Model file for the job. Use its own axes, mm. Give positions to 0.01 mm unless a question says otherwise; leave off trailing zeros. Loops run counter-clockwise (first coordinate to the right, second up) from the corner with the lowest first, then second, coordinate; pieces in that order, holes last. Notation, with made-up numbers: (1, 81.25) -> (18, 81.25) arc R18 ccw to (18, 112.25) -> close; hole circle Ø11 at (88.25, 5.25). An arc over 180 degrees is marked (long way). Use CSV: the item, a comma, the result in double quotes. Start each with the question number.
(1) Cut at B-B on y = 0. Write the cut outline in (x, z).
(2) Cut at D-D on x = 57. Write the cut outline in (y, z), then the cut area to 3 significant figures.
(3) Cut at C-C on y = -34.5. Write the cut outline in (x, z).
(4) Cut at A-A on x = 28. Write the cut outline in (y, z).
(5) Flat gauge pins, fed straight in: pin 1 (2 mm diameter, centred on x = 54, y = -12, fed in from -Z); pin 2 (3.5 mm diameter, centred on x = 57, y = 27.5, fed in from -Z). Where does each tip first touch, or does it go through?
(6) Drill centre lines: probe 1 along Y at (x, z) = (36, 2.25); probe 2 along Y at (x, z) = (57, 1.1); probe 3 along Y at (x, z) = (24, 1.55). Where is each one in solid material? Low to high.
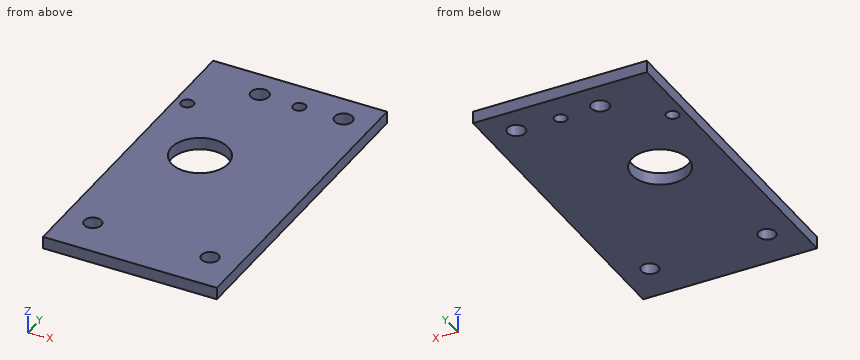
from build123d import *

# Parameters (mm, degrees)
SKETCH_1_W                = 40
SKETCH_1_H                = 29
EXTRUDE_1_DEPTH           = 3
CUT_EXTRUDE_1_DEPTH       = 3
SKETCH_3_W                = 40
SKETCH_3_H                = 3
EXTRUDE_2_DEPTH           = 10
SKETCH_4_W                = 40
SKETCH_4_H                = 3
EXTRUDE_3_DEPTH           = 10
SKETCH_6_W                = 3
SKETCH_6_H                = 49
EXTRUDE_5_DEPTH           = 42
SKETCH_8_W                = 3
SKETCH_8_H                = 49
EXTRUDE_6_DEPTH           = 2
SKETCH_9_W                = 3
SKETCH_9_H                = 49
EXTRUDE_7_DEPTH           = 2
SKETCH_10_W               = 86
SKETCH_10_H               = 3
EXTRUDE_8_DEPTH           = 10
SKETCH_11_W               = 86
SKETCH_11_H               = 3
EXTRUDE_9_DEPTH           = 10
SKETCH_7_R                = 7
CUT_EXTRUDE_4_DEPTH       = 10
SKETCH_14_W               = 3
SKETCH_14_H               = 69
CUT_EXTRUDE_5_DEPTH       = 43
SKETCH_17_W               = 43
SKETCH_17_H               = 3
EXTRUDE_10_DEPTH          = 20
SKETCH_18_R               = 2.1
CUT_EXTRUDE_6_DEPTH       = 10
SKETCH_20_W               = 43
SKETCH_20_H               = 3
EXTRUDE_11_DEPTH          = 10
SKETCH_21_W               = 43
SKETCH_21_H               = 3
CUT_EXTRUDE_7_DEPTH       = 20
SKETCH_24_R               = 2.2
CUT_EXTRUDE_8_DEPTH       = 30
SKETCH_25_R               = 1.55
CUT_EXTRUDE_11_DEPTH      = 1
CUT_EXTRUDE_11_DEPTH_BACK = 4


with BuildPart() as part:
    # ｽｹｯﾁ1 → ﾎﾞｽ - 押し出し1 (new body)
    with BuildSketch(Plane.XY):
        Rectangle(SKETCH_1_W, SKETCH_1_H)
    extrude(amount=EXTRUDE_1_DEPTH)

    # ｽｹｯﾁ2 → ｶｯﾄ - 押し出し1 (cut)
    with BuildSketch(Plane.XY.offset(3)):
        with BuildLine():
            ThreePointArc((-14.4, 10.5), (-15.01507576, 11.98492424), (-16.5, 12.6))
            Line((-16.5, 12.6), (-16.5, 10.5))
            Line((-16.5, 10.5), (-18.6, 10.5))
            ThreePointArc((-18.6, 10.5), (-16.5, 8.4), (-14.4, 10.5))
        make_face()
        with BuildLine():
            Line((-16.5, 10.5), (-16.5, 12.6))
            ThreePointArc((-16.5, 12.6), (-17.98492424, 11.98492424), (-18.6, 10.5))
            Line((-18.6, 10.5), (-16.5, 10.5))
        make_face()
        with BuildLine():
            ThreePointArc((-18.6, -10.5), (-17.98492424, -11.98492424), (-16.5, -12.6))
            Line((-16.5, -12.6), (-16.5, -10.5))
            Line((-16.5, -10.5), (-18.6, -10.5))
        make_face()
        with BuildLine():
            Line((-16.5, -10.5), (-16.5, -12.6))
            ThreePointArc((-16.5, -12.6), (-15.01507576, -11.98492424), (-14.4, -10.5))
            ThreePointArc((-14.4, -10.5), (-16.5, -8.4), (-18.6, -10.5))
            Line((-18.6, -10.5), (-16.5, -10.5))
        make_face()
        with BuildLine():
            ThreePointArc((18.6, -10.5), (15.01507576, -9.01507576), (16.5, -12.6))
            Line((16.5, -12.6), (16.5, -10.5))
            Line((16.5, -10.5), (18.6, -10.5))
        make_face()
        with BuildLine():
            Line((16.5, -10.5), (16.5, -12.6))
            ThreePointArc((16.5, -12.6), (17.98492424, -11.98492424), (18.6, -10.5))
            Line((18.6, -10.5), (16.5, -10.5))
        make_face()
        with BuildLine():
            ThreePointArc((18.6, 10.5), (17.98492424, 11.98492424), (16.5, 12.6))
            Line((16.5, 12.6), (16.5, 10.5))
            Line((16.5, 10.5), (18.6, 10.5))
        make_face()
        with BuildLine():
            Line((16.5, 10.5), (16.5, 12.6))
            ThreePointArc((16.5, 12.6), (15.01507576, 9.01507576), (18.6, 10.5))
            Line((18.6, 10.5), (16.5, 10.5))
        make_face()
    extrude(amount=-CUT_EXTRUDE_1_DEPTH, mode=Mode.SUBTRACT)

    # ｽｹｯﾁ3 → ﾎﾞｽ - 押し出し2 (add)
    with BuildSketch(Plane.XZ.offset(14.5)):
        with Locations((0, 1.5)):
            Rectangle(SKETCH_3_W, SKETCH_3_H)
    extrude(amount=EXTRUDE_2_DEPTH)

    # ｽｹｯﾁ4 → ﾎﾞｽ - 押し出し3 (add)
    with BuildSketch(Plane(origin=(0, 14.5, 0), x_dir=(1, 0, 0), z_dir=(0, 1, 0))):
        with Locations((0, -1.5)):
            Rectangle(SKETCH_4_W, SKETCH_4_H)
    extrude(amount=EXTRUDE_3_DEPTH)

    # ｽｹｯﾁ6 → ﾎﾞｽ - 押し出し5 (add)
    with BuildSketch(Plane(origin=(20, 0, 0), x_dir=(0, 0, -1), z_dir=(1, 0, 0))):
        with Locations((-1.5, 0)):
            Rectangle(SKETCH_6_W, SKETCH_6_H)
    extrude(amount=EXTRUDE_5_DEPTH)

    # ｽｹｯﾁ8 → ﾎﾞｽ - 押し出し6 (add)
    with BuildSketch(Plane.ZY.offset(20)):
        with Locations((1.5, 0)):
            Rectangle(SKETCH_8_W, SKETCH_8_H)
    extrude(amount=EXTRUDE_6_DEPTH)

    # ｽｹｯﾁ9 → ﾎﾞｽ - 押し出し7 (add)
    with BuildSketch(Plane(origin=(62, 0, 0), x_dir=(0, 0, -1), z_dir=(1, 0, 0))):
        with Locations((-1.5, 0)):
            Rectangle(SKETCH_9_W, SKETCH_9_H)
    extrude(amount=EXTRUDE_7_DEPTH)

    # ｽｹｯﾁ10 → ﾎﾞｽ - 押し出し8 (add)
    with BuildSketch(Plane.XZ.offset(24.5)):
        with Locations((21, 1.5)):
            Rectangle(SKETCH_10_W, SKETCH_10_H)
    extrude(amount=EXTRUDE_8_DEPTH)

    # ｽｹｯﾁ11 → ﾎﾞｽ - 押し出し9 (add)
    with BuildSketch(Plane(origin=(0, 24.5, 0), x_dir=(1, 0, 0), z_dir=(0, 1, 0))):
        with Locations((21, -1.5)):
            Rectangle(SKETCH_11_W, SKETCH_11_H)
    extrude(amount=EXTRUDE_9_DEPTH)

    # ｽｹｯﾁ7 → ｶｯﾄ - 押し出し4 (cut)
    with BuildSketch(Plane.XY.offset(3)):
        with Locations((36.10579786, 0)):
            Circle(SKETCH_7_R)
    extrude(amount=-CUT_EXTRUDE_4_DEPTH, mode=Mode.SUBTRACT)

    # ｽｹｯﾁ14 → ｶｯﾄ - 押し出し5 (cut)
    with BuildSketch(Plane.ZY.offset(22)):
        with Locations((1.5, 0)):
            Rectangle(SKETCH_14_W, SKETCH_14_H)
    extrude(amount=-CUT_EXTRUDE_5_DEPTH, mode=Mode.SUBTRACT)

    # ｽｹｯﾁ17 → ﾎﾞｽ - 押し出し10 (add)
    with BuildSketch(Plane.XZ.offset(34.5)):
        with Locations((42.5, 1.5)):
            Rectangle(SKETCH_17_W, SKETCH_17_H)
    extrude(amount=EXTRUDE_10_DEPTH)

    # ｽｹｯﾁ18 → ｶｯﾄ - 押し出し6 (cut)
    with BuildSketch(Plane.XY.offset(3)):
        with Locations((28, -34.5)):
            Circle(SKETCH_18_R)
        with Locations((57, -34.5)):
            Circle(SKETCH_18_R)
    extrude(amount=-CUT_EXTRUDE_6_DEPTH, mode=Mode.SUBTRACT)

    # ｽｹｯﾁ20 → ﾎﾞｽ - 押し出し11 (add)
    with BuildSketch(Plane.XZ.offset(54.5)):
        with Locations((42.5, 1.5)):
            Rectangle(SKETCH_20_W, SKETCH_20_H)
    extrude(amount=EXTRUDE_11_DEPTH)

    # ｽｹｯﾁ21 → ｶｯﾄ - 押し出し7 (cut)
    with BuildSketch(Plane.XZ.offset(64.5)):
        with Locations((42.5, 1.5)):
            Rectangle(SKETCH_21_W, SKETCH_21_H)
    extrude(amount=-CUT_EXTRUDE_7_DEPTH, mode=Mode.SUBTRACT)

    # ｽｹｯﾁ24 → ｶｯﾄ - 押し出し8 (cut)
    with BuildSketch(Plane(origin=(0, 0, 0), x_dir=(-1, 0, 0), z_dir=(0, 0, -1))):
        with Locations((-36.27, 27.5)):
            Circle(SKETCH_24_R)
        with Locations((-57, 27.5)):
            Circle(SKETCH_24_R)
    extrude(amount=-CUT_EXTRUDE_8_DEPTH, mode=Mode.SUBTRACT)

    # ｽｹｯﾁ25 → ｶｯﾄ - 押し出し11 (cut, two sides)
    with BuildSketch(Plane(origin=(0, 0, 0), x_dir=(-1, 0, 0), z_dir=(0, 0, -1))) as cut_extrude_11_sk:
        with Locations((-24, 16.905537109)):
            Circle(SKETCH_25_R)
        with Locations((-46.2, 27.205537109)):
            Circle(SKETCH_25_R)
    extrude(amount=CUT_EXTRUDE_11_DEPTH, mode=Mode.SUBTRACT)
    extrude(cut_extrude_11_sk.sketch, amount=-CUT_EXTRUDE_11_DEPTH_BACK, mode=Mode.SUBTRACT)


solid = part.part
Check result:
1,outline,"(21, 0) -> (29.11, 0) -> (29.11, 3) -> (21, 3) -> close; (43.11, 0) -> (64, 0) -> (64, 3) -> (43.11, 3) -> close"
2,outline,"(-44.5, 0) -> (-36.6, 0) -> (-36.6, 3) -> (-44.5, 3) -> close; (-32.4, 0) -> (25.3, 0) -> (25.3, 3) -> (-32.4, 3) -> close; (29.7, 0) -> (34.5, 0) -> (34.5, 3) -> (29.7, 3) -> close"
2,area,"211 mm²"
3,outline,"(21, 0) -> (25.9, 0) -> (25.9, 3) -> (21, 3) -> close; (30.1, 0) -> (54.9, 0) -> (54.9, 3) -> (30.1, 3) -> close; (59.1, 0) -> (64, 0) -> (64, 3) -> (59.1, 3) -> close"
4,outline,"(-44.5, 0) -> (-36.6, 0) -> (-36.6, 3) -> (-44.5, 3) -> close; (-32.4, 0) -> (34.5, 0) -> (34.5, 3) -> (-32.4, 3) -> close"
5,pin 1,"z = 0"
5,pin 2,"through"
6,probe 1,"-44.5 to -7, 7 to 25.32, 29.68 to 34.5"
6,probe 2,"-44.5 to -36.6, -32.4 to 25.3, 29.7 to 34.5"
6,probe 3,"-44.5 to 15.36, 18.46 to 34.5"
